Here's how the part is built. I have some questions about the finished solid (model axes, mm). Face numbers are marked on the shaded views. A direction names the side the tool comes from. Give positions to 0.01 mm unless a question says otherwise; leave off trailing zeros. Loops run counter-clockwise (first coordinate to the right, second up) from the corner with the lowest first, then second, coordinate; pieces in that order, holes last. Notation, with made-up numbers: (76, 64.25) - (91, 64.25) arc R20 cw to (91, 100.25) - close; hole circle Ø6 at (35, 51.5). An arc over 180 degrees is marked (long way). Return JSON: item names as keys, results as strings. Group by question number.
(1) If we mould it in two halves opening along X, with no side actions, what happens to the marked faces 1, 2, 3 and 4? For each: released by +X, released by -X, zero draft, split by the parting line, or undercut.
(2) If we section it at D-D (z = 34): Please give me the cut outline in (x, y), then the cut area to 3 significant figures.
(3) I need wall thicknesses on probe 1 along Z at (x, y) = (36, 40.5); probe 2 along X at (y, z) = (24, 5); probe 3 along Y at (x, z) = (33, 36.5). Which ranges of each line are inside material? Lowest first, please. Write a range as [from, to].
(4) If we section it at B-B (z = 9): Please give me the cut outline in (x, y) (3 decimals).
(5) For P1, Ø3.5, axis at x = 25.5, y = 31.5, coming from the +Z side; P2, Ø5.5, axis at x = 37.5, y = 28, coming from the -Z side; P3, Ø7, axis at y = 16.5, z = 10.5, coming from the -X side; P4, Ø8, axis at x = 18.5, y = 14.5, coming from the +Z side, each with a flat end and sliding along its axis, tell me the tip position at first contact or that it passes through.
(6) On a 3-axis mill with a long thin cutter (end or side, diameter ignored), from which of +Z, -Z, +X, -X, +Y, -Y can I reach the whole of each face in a straight line? I mean the marked faces 5, 6 and 7. Say none if no direction works.
(7) If we section it at A-A (x = 25): State how many separate pieces and enclosed holes the cut face has, then the cut area to 3 significant figures.
(8) If we section it at C-C (y = 29): Please give me the cut outline in (x, z).
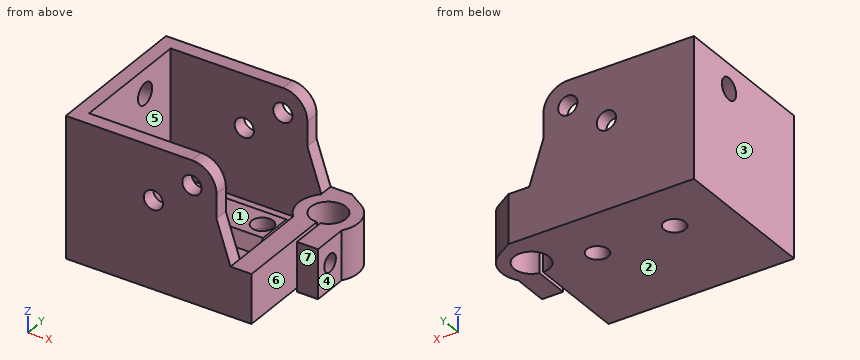
```python
from build123d import *

# Parameters (mm, degrees)
F0_W           = 53
F0_H           = 43
F1_DEPTH       = 5
F3_DEPTH       = 9
F3_DEPTH_BACK  = 5
F4_DEPTH       = 25
F6_DEPTH       = 35
F7_R           = 2.75
F8_DEPTH       = 43.001
F10_DEPTH      = 3
F10_DEPTH_BACK = 6
F11_R          = 2.5
F12_DEPTH      = 25
F13_W          = 37.7532099868
F13_H          = 10
F14_DEPTH      = 3
F15_R          = 3.05
F16_DEPTH      = 25
F16_DEPTH_BACK = 25
F17_SIZE       = 2.99999
F18_R          = 3.05
F19_DEPTH      = 25


# Not quite as in the source:
# - a fillet or chamfer is up to 0.001 mm smaller than in the source, because OpenCascade refuses the exact size


with BuildPart() as f1:
    # F0 (on Top) → F1 (new body)
    with BuildSketch(Plane.XY):
        with Locations((26.5, 21.5)):
            Rectangle(F0_W, F0_H)
    extrude(amount=F1_DEPTH)

    # F2 (on face) → F3 (join, two sides)
    with BuildSketch(Plane.XY.offset(5)) as f3_sk:
        with BuildLine():
            Line((47, 0), (53, 0))
            Line((53, 0), (53, 24.5))
            Line((53, 24.5), (53, 28))
            ThreePointArc((53, 28), (52.49745519, 37.974680765), (54, 28.1010205144))
            Line((54, 28.1010205144), (54, 24.5590284919))
            Line((54, 24.5590284919), (54, 18))
            Line((54, 18), (60, 18))
            Line((60, 18), (60, 25.8046761155))
            Line((60, 25.8046761155), (60, 28.1781746195))
            ThreePointArc((60, 28.1781746195), (61.3195930877, 34.7419445616), (57.477652845, 40.225))
            Line((57.477652845, 40.225), (53, 43))
            Line((53, 43), (47, 43))
            Line((47, 43), (46.9, 43))
            Line((46.9, 43), (46.9, 38.9194594348))
            ThreePointArc((46.9, 38.9194594348), (44.5002980841, 32.9288147474), (47, 26.9792027106))
            Line((47, 26.9792027106), (47, 0))
        make_face()
    extrude(amount=F3_DEPTH)
    extrude(f3_sk.sketch, amount=-F3_DEPTH_BACK)

    # F2 (on face) → F4 (cut)
    with BuildSketch(Plane.XY.offset(5)):
        with BuildLine():
            ThreePointArc((53, 38), (48, 33), (53, 28))
            Line((53, 28), (53, 28.1010205144))
            Line((53, 28.1010205144), (53, 38))
        make_face()
    extrude(amount=-F4_DEPTH, mode=Mode.SUBTRACT)

    # F5 (on face) → F6 (join)
    with BuildSketch(Plane.XY.offset(5)):
        Polygon((0, 43), (0, 0), (47, 0), (47, 4.00000019), (4.00000019, 4.00000019), (4.00000019, 38.99999981), (46.9636693597, 38.99999981), (46.9636693597, 43), align=None)
    extrude(amount=F6_DEPTH)

    # F7 (on face) → F8 (cut, through all)
    with BuildSketch(Plane.XZ):
        with Locations((36, 33)):
            Circle(F7_R)
        with Locations((25, 25)):
            Circle(F7_R)
        with BuildLine():
            ThreePointArc((36, 40), (40.9497474683, 37.9497474683), (43, 33))
            Line((43, 33), (43, 26))
            Line((43, 26), (47, 14))
            Line((47, 14), (47, 40))
            Line((47, 40), (36, 40))
        make_face()
    extrude(amount=-F8_DEPTH, mode=Mode.SUBTRACT)

    # F9 (on face) → F10 (cut, two sides)
    with BuildSketch(Plane(origin=(47, 0, 0), x_dir=(0, -1, 0), z_dir=(-1, 0, 0))) as f10_sk:
        Polygon((-18.9281746195, 5.0462613559), (-18.9281746195, 9.9537386441), (-23.1781746195, 12.4074772881), (-27.4281746195, 9.9537386441), (-27.4281746195, 5.0462613559), (-23.1781746195, 2.5925227119), align=None)
    extrude(amount=-F10_DEPTH, mode=Mode.SUBTRACT)
    extrude(f10_sk.sketch, amount=F10_DEPTH_BACK, mode=Mode.SUBTRACT)

    # F11 (on face) → F12 (cut)
    with BuildSketch(Plane.YZ.offset(60)):
        with Locations((23.1781746195, 7.5)):
            Circle(F11_R)
    extrude(amount=-F12_DEPTH, mode=Mode.SUBTRACT)

    # F13 (on face) → F14 (join)
    with BuildSketch(Plane.XY.offset(5)):
        with Locations((22.1233950066, 28)):
            Rectangle(F13_W, F13_H)
    extrude(amount=F14_DEPTH)

    # F15 (on face) → F16 (cut, two sides)
    with BuildSketch(Plane.XY.offset(5)) as f16_sk:
        with Locations((15.5, 28)):
            Circle(F15_R)
        with Locations((37.5, 28)):
            Circle(F15_R)
    extrude(amount=-F16_DEPTH, mode=Mode.SUBTRACT)
    extrude(f16_sk.sketch, amount=F16_DEPTH_BACK, mode=Mode.SUBTRACT)

    # F17 (size 3 in the source; OpenCascade refuses exactly that, so slightly less here)
    f17_edges = [f1.edges().sort_by_distance(p)[0] for p in [
        (22.5, 23, 5),
        (22.5, 33, 5),
    ]]
    chamfer(f17_edges, length=F17_SIZE)

    # F18 (on face) → F19 (cut)
    with BuildSketch(Plane(origin=(0, 0, 0), x_dir=(0, -1, 0), z_dir=(-1, 0, 0))):
        with Locations((-28, 33)):
            Circle(F18_R)
    extrude(amount=-F19_DEPTH, mode=Mode.SUBTRACT)


solid = f1.part
```
Values:
{
 "1": {"face 1": "undercut", "face 2": "zero draft", "face 3": "released by -X", "face 4": "released by +X"},
 "2": {"outline": "(0, 0) - (33.44, 0) - (33.44, 4) - (4, 4) - (4, 25.12) - (0, 25.12) - close; (0, 30.88) - (4, 30.88) - (4, 39) - (33.44, 39) - (33.44, 43) - (0, 43) - close; (38.56, 0) - (42.93, 0) - (42.93, 4) - (38.56, 4) - close; (38.56, 39) - (42.93, 39) - (42.93, 43) - (38.56, 43) - close", "area": "419 mm2"},
 "3": {"probe 1": "[0, 30.25], [35.75, 40]", "probe 2": "[0, 41], [50, 53], [54, 60]", "probe 3": "[0, 4], [39, 43]"},
 "4": {"outline": "(0, 0) - (53, 0) - (53, 21.178) - (50, 21.178) - (50, 18.928) - (47, 18.928) - (47, 4) - (4, 4) - (4, 39) - (46.9, 39) - (46.9, 38.919) arc R8.5 ccw to (46.581, 27.428) - (50, 27.428) - (50, 25.178) - (53, 25.178) - (53, 28) arc R5 cw (long way) to (54, 28.101) - (54, 25.178) - (60, 25.178) - (60, 28.178) arc R8.5 ccw to (57.478, 40.225) - (53, 43) - (0, 43) - close; (54, 18) - (60, 18) - (60, 21.178) - (54, 21.178) - close"},
 "5": {"P1": "z = 8", "P2": "through", "P3": "x = 0", "P4": "z = 5"},
 "6": {"face 5": "+Z", "face 6": "+Z, -Z, -Y", "face 7": "+Z, -Z, +X, -Y"},
 "7": {"separate pieces": "3", "enclosed holes": "0", "area": "490 mm2"},
 "8": {"outline": "(0, 0) - (12.62, 0) - (12.62, 8) - (4, 8) - (4, 30.12) - (0, 30.12) - close; (0, 35.88) - (4, 35.88) - (4, 40) - (0, 40) - close; (18.38, 0) - (34.62, 0) - (34.62, 8) - (18.38, 8) - close; (40.38, 0) - (50, 0) - (50, 14) - (45.5, 14) - (45.5, 5) - (41, 5) - (41, 8) - (40.38, 8) - close; (56, 0) - (60.5, 0) - (60.5, 14) - (56, 14) - close"}
}
